For this review, take the finished solid that the model builds, in its own axes (mm). A direction names the side the tool comes from. Give positions to 0.01 mm unless a question says otherwise; leave off trailing zeros. Order: outer loops, then holes, each group sorted by start corner. A loop starts at its lowest first (then second) coordinate and runs counter-clockwise, first axis right, second up. Notation, with made-up numbers: (63, 54) - (109, 54) arc R14 cw to (109, 70) - close; hole circle Ø10 at (46, 50.5). An arc over 180 degrees is marked (long way). Use a Markdown table: item, result. Add a question column.
1) Clearance check with flat-ended pins moving along their axes: P1, Ø2, axis at x = -12, y = 0, coming from the -Z side; P2, Ø1, axis at y = 11, z = 1, coming from the -X side; P3, Ø1, axis at x = 3, y = 3, coming from the +Z side; P4, Ø1.5, axis at x = 13, z = 4.5, coming from the -Y side. State where each tip first meets the part, or that it passes through.
2) Machinability: for faces 1 (the face through (-1.18, 0.16, 2.45)), 2 (the face through (0, 0, 0)), which of the approach directions +Z, -Z, +X, -X, +Y, -Y give a long, thin tool a straight path to every point of the face, cutting with its end or side? Answer none if there is none.
3) Mouldability with a two-part tool opening along X and no side actions: class faces 3 (the face through (0, 0, 9)), 4 (the face through (13.025, -5.4, 1.711)), 5 (the face through (-11.67, 0.25, 6.15)) as released by +X, released by -X, zero draft, split by the parting line, or undercut.
4) Wall thickness on L1, parallel to X at y = -6.5, z = 4.75; L2, parallel to X at y = 9, z = 4.5; L3, parallel to Y at x = -8, z = 7.5: over which ranges is each line inside the solid? List them lowest first.
5) We need section B-B on z = 4.5. Give the number of separate pieces and of enclosed holes in the cut face, then the cut area to 3 significant figures.
6) We need section A-A on z = 2.5. Write out the cut boundary in (x, y), then the cut area to 3 significant figures.
```python
from build123d import *

# Parameters (mm, degrees)
F3_DEPTH = 0.75
F4_R     = 1.5
F5_R     = 5


with BuildPart() as f1:
    # F0 (on Front) → F1 (revolve)
    with BuildSketch(Plane.XZ):
        Polygon((0, 2), (0, 0), (14.1, 0), (14.1, 6), (17, 8), (17, 9), (15.8079127569, 9), (11.4579127569, 6), (11.4579127569, 2), align=None)
    revolve(axis=Axis((0, 0, 4.5), (0, 0, 1)))

    # F2 (on Right) → F3 (join, symmetric)
    with BuildSketch(Plane.YZ):
        Polygon((16, 9), (-16, 9), (-16, 8), (-13.1, 6), (-13.1, 0), (13.1, 0), (13.1, 6), (16, 8), align=None)
    extrude(amount=F3_DEPTH, both=True)

    # F4
    f4_edges = [f1.edges().sort_by_distance(p)[0] for p in [
        (-11.457913, 0, 2),
        (0.75, 0, 2),
        (11.457913, 0, 2),
        (-0.75, 0, 2),
    ]]
    fillet(f4_edges, radius=F4_R)

    # F5
    f5_edges = [f1.edges().sort_by_distance(p)[0] for p in [
        (-14.1, 0, 6),
    ]]
    fillet(f5_edges, radius=F5_R)


solid = f1.part
```
Checked values:
| question | item | result |
|---|---|---|
| 1 | P1 | z = 0 |
| 1 | P2 | x = -9.41 |
| 1 | P3 | z = 2 |
| 1 | P4 | y = -7.29 |
| 2 | face 1 | +Z |
| 2 | face 2 | -Z, +X, -X, +Y, -Y |
| 3 | face 3 | zero draft |
| 3 | face 4 | split by the parting line |
| 3 | face 5 | undercut |
| 4 | L1 | -12.73 to -9.44, -0.75 to 0.75, 9.44 to 12.73 |
| 4 | L2 | -11.02 to -7.09, -0.75 to 0.75, 7.09 to 11.02 |
| 4 | L3 | -14.17 to -11.04, 11.04 to 14.17 |
| 5 | separate pieces | 1 |
| 5 | enclosed holes | 2 |
| 5 | area | 258 mm² |
| 6 | outline | circle Ø28.2 at (0, 0); hole (-1.13, -11.02) - (-1.13, 11.02) arc R11.08 ccw to start; hole (1.13, -11.02) arc R11.08 ccw to (1.13, 11.02) - close |
| 6 | area | 289 mm² |
